from build123d import *

# Parameters (mm, degrees)
SKETCH_2_W          = 94.97478029
SKETCH_2_H          = 42.97467615
SKETCH_2_W_2        = 90.97478029
SKETCH_2_H_2        = 38.97467615
EXTRUDE_1_DEPTH     = 5
SKETCH_3_W          = 94.97478029
SKETCH_3_H          = 42.97467615
EXTRUDE_2_DEPTH     = 3.4
SKETCH_4_W          = 43.8
SKETCH_4_H          = 35.9
CUT_EXTRUDE_1_DEPTH = 0.4
FILLET_1_R          = 4.5
CUT_EXTRUDE_2_DEPTH = 2.4
CUT_EXTRUDE_3_DEPTH = 0.6
FILLET_2_R          = 4
FILLET_3_R          = 0.5
CHAMFER_1_SIZE      = 0.5


with BuildPart() as part:
    # 草图2 → 凸台-拉伸1 (new body)
    with BuildSketch(Plane.XY):
        with Locations((45.00009017, -19.0000381)):
            Rectangle(SKETCH_2_W, SKETCH_2_H)
        with Locations((45.00009017, -19.0000381)):
            Rectangle(SKETCH_2_W_2, SKETCH_2_H_2, mode=Mode.SUBTRACT)
    extrude(amount=EXTRUDE_1_DEPTH)

    # 草图3 → 凸台-拉伸2 (add)
    with BuildSketch(Plane.XY.offset(5)):
        with Locations((45.00009017, -19.0000381)):
            Rectangle(SKETCH_3_W, SKETCH_3_H)
    extrude(amount=EXTRUDE_2_DEPTH)

    # 草图4 → 切除-拉伸1 (cut)
    with BuildSketch(Plane.XY.offset(8.4)):
        with Locations((45.012700025, -19.012700025)):
            Rectangle(SKETCH_4_W, SKETCH_4_H)
    extrude(amount=-CUT_EXTRUDE_1_DEPTH, mode=Mode.SUBTRACT)

    # 圆角1
    fillet_1_edges = [part.edges().sort_by_distance(p)[0] for p in [
        (23.112700025, -36.962700025, 8.2),
        (23.112700025, -1.062700025, 8.2),
        (66.912700025, -1.062700025, 8.2),
        (66.912700025, -36.962700025, 8.2),
    ]]
    fillet(fillet_1_edges, radius=FILLET_1_R)

    # 草图5 → 切除-拉伸2 (cut)
    with BuildSketch(Plane.XY.offset(8)):
        Polygon((25.112700025, -3.062700025), (64.612700025, -3.062700025), (64.612700025, -11.062700025), (66.112700025, -11.062700025), (66.112700025, -24.962700025), (64.612700025, -24.962700025), (64.612700025, -34.962700025), (25.112700025, -34.962700025), align=None)
    extrude(amount=-CUT_EXTRUDE_2_DEPTH, mode=Mode.SUBTRACT)

    # 草图6 → 切除-拉伸3 (cut)
    with BuildSketch(Plane.XY.offset(5.6)):
        Polygon((35.112700025, -3.062700025), (64.612700025, -3.062700025), (64.612700025, -11.062700025), (66.112700025, -11.062700025), (66.112700025, -24.962700025), (64.612700025, -24.962700025), (64.612700025, -34.962700025), (35.112700025, -34.962700025), align=None)
    extrude(amount=-CUT_EXTRUDE_3_DEPTH, mode=Mode.SUBTRACT)

    # 圆角2
    fillet_2_edges = [part.edges().sort_by_distance(p)[0] for p in [
        (25.112700025, -34.962700025, 6.8),
        (25.112700025, -3.062700025, 6.8),
        (64.612700025, -3.062700025, 6.5),
        (64.612700025, -34.962700025, 6.5),
    ]]
    fillet(fillet_2_edges, radius=FILLET_2_R)

    # 圆角3
    fillet_3_edges = [part.edges().sort_by_distance(p)[0] for p in [
        (35.112700025, -34.962700025, 5.3),
        (35.112700025, -3.062700025, 5.3),
        (64.612700025, -11.062700025, 6.5),
        (66.112700025, -11.062700025, 6.5),
        (66.112700025, -24.962700025, 6.5),
        (64.612700025, -24.962700025, 6.5),
    ]]
    fillet(fillet_3_edges, radius=FILLET_3_R)

    # 倒角1
    chamfer_1_edges = [part.edges().sort_by_distance(p)[0] for p in [
        (64.612700025, -28.212700025, 8),
        (44.862700025, -34.962700025, 8),
        (25.112700025, -19.012700025, 8),
        (44.862700025, -3.062700025, 8),
        (63.44112715, -33.79112715, 8),
        (26.284272901, -33.79112715, 8),
        (63.44112715, -4.234272901, 8),
        (26.284272901, -4.234272901, 8),
        (66.112700025, -18.012700025, 8),
        (65.362700025, -24.962700025, 8),
        (65.362700025, -11.062700025, 8),
        (64.612700025, -8.812700025, 8),
        (64.759146635, -25.109146635, 8),
        (64.759146635, -10.916253416, 8),
        (65.966253416, -24.816253416, 8),
        (65.966253416, -11.209146635, 8),
    ]]
    chamfer(chamfer_1_edges, length=CHAMFER_1_SIZE - 0.0001)  # a hair under: the kernel refuses the full size


solid = part.part
Geometry: final body of the model. Coordinates: model frame, mm. A direction names the side the tool comes from. Round coordinates to 2 decimals unless told otherwise and drop trailing zeros. Loops run counter-clockwise (first coordinate to the right, second up) from the corner with the lowest first, then second, coordinate; pieces in that order, holes last.
Q1. Material intervals for L1, parallel to X at y = -18, z = 5.25; L2, parallel to X at y = -12.5, z = 5.75; L3, parallel to Y at x = 26, z = 1.5, sorted ascending.
Q2. Section C-C on x = 58. Return loops of the section in (y, z), plus the area to 3 significant figures.
Q3. Pull-direction query (Y, two-part tool) for faces 4 (the flat face through (45, -34.963, 6)), 5 (the flat face through (44, 2.487, 4)), 6 (the flat face through (92.487, -19, 4)), 7 (the flat face through (44, -40.487, 4)); classes: released by +Y, released by -Y, zero draft, split by the parting line, or undercut.
Q4. Access query for faces 1 (the flat face through (64.613, -9, 6)), 2 (the flat face through (34, -19, 5)), 3 (the conical face through (63.569, -33.855, 7.635)). Directions: +Z, -Z, +X, -X, +Y, -Y. A direction counts if a zero-diameter tool reaches every point of the face in a straight line with its end or side. Return the directions, or none.
Q5. Pin query (flat end, axial travel): P1, Ø3, axis at x = 34.5, y = -31.5, coming from the +Z side. Return the tip coordinate at first contact, or that it passes through.
Q6. Section D-D on x = 4. Return loops of the section in (y, z).
Q7. Section B-B on z = 1.5. Return loops of the section in (x, y), plus the area to 3 significant figures.
Q8. Section A-A on y = -9.5. Return loops of the section in (x, z).
Evaluation:
1. L1: x = -2.49 to 35.11, 66.11 to 92.49
1. L2: x = -2.49 to 25.11, 66.11 to 92.49
1. L3: y = -40.49 to -38.49, 0.49 to 2.49
2. outline: (-40.49, 0) - (-38.49, 0) - (-38.49, 5) - (-34.96, 5) - (-34.96, 7.5) - (-35.46, 8) - (-36.96, 8) - (-36.96, 8.4) - (-40.49, 8.4) - close; (-3.06, 5) - (0.49, 5) - (0.49, 0) - (2.49, 0) - (2.49, 8.4) - (-1.06, 8.4) - (-1.06, 8) - (-2.56, 8) - (-3.06, 7.5) - close
2. area: 55.8 mm2
3. face 4: undercut
3. face 5: released by +Y
3. face 6: zero draft
3. face 7: released by -Y
4. face 1: +Z, -Z
4. face 2: -Z
4. face 3: +Z
5. P1: stops at z = 5.6
6. outline: (-40.49, 0) - (-38.49, 0) - (-38.49, 5) - (0.49, 5) - (0.49, 0) - (2.49, 0) - (2.49, 8.4) - (-40.49, 8.4) - close
7. outline: (-2.49, -40.49) - (92.49, -40.49) - (92.49, 2.49) - (-2.49, 2.49) - close; hole (-0.49, -38.49) - (90.49, -38.49) - (90.49, 0.49) - (-0.49, 0.49) - close
7. area: 536 mm2
8. outline: (-2.49, 0) - (-0.49, 0) - (-0.49, 5) - (35.11, 5) - (35.11, 5.6) - (25.11, 5.6) - (25.11, 7.5) - (24.61, 8) - (23.11, 8) - (23.11, 8.4) - (-2.49, 8.4) - close; (64.61, 5) - (90.49, 5) - (90.49, 0) - (92.49, 0) - (92.49, 8.4) - (66.91, 8.4) - (66.91, 8) - (65.11, 8) - (64.61, 7.5) - close
